```python
from build123d import *

# Parameters (mm, degrees)
F2_W     = 20
F2_H     = 20
F3_DEPTH = 2
F4_W     = 20
F4_H     = 20
F5_DEPTH = 18
F6_R     = 1.85
F7_DEPTH = 10


with BuildPart() as f3:
    # F2 (on Top) → F3 (new body)
    with BuildSketch(Plane.XY):
        with Locations((10, -10)):
            Rectangle(F2_W, F2_H)
    extrude(amount=F3_DEPTH)

    # F4 (on face) → F5 (join)
    with BuildSketch(Plane.XY.offset(2)):
        with Locations((10, -10)):
            Rectangle(F4_W, F4_H)
        Polygon((2, -6.06223871), (2, -2), (6.06223871, -2), (13.93776129, -2), (18, -2), (18, -6.06223871), (18, -13.93776129), (18, -18), (13.93776129, -18), (6.06223871, -18), (2, -18), (2, -13.93776129), align=None, mode=Mode.SUBTRACT)
        Polygon((6.06223871, -2), (2, -2), (2, -6.06223871), align=None)
        Polygon((18, -2), (13.93776129, -2), (18, -6.06223871), align=None)
        Polygon((18, -18), (18, -13.93776129), (13.93776129, -18), align=None)
        Polygon((6.06223871, -18), (2, -13.93776129), (2, -18), align=None)
    extrude(amount=F5_DEPTH)

    # F6 (on face) → F7 (cut)
    with BuildSketch(Plane.XY.offset(20)):
        with Locations((2.1344347065, -2.3655652935)):
            Circle(F6_R)
        with Locations((17.6344347065, -2.3655652935)):
            Circle(F6_R)
        with Locations((17.6344347065, -17.3655652935)):
            Circle(F6_R)
        with Locations((2.1344347065, -17.3655652935)):
            Circle(F6_R)
    extrude(amount=-F7_DEPTH, mode=Mode.SUBTRACT)


solid = f3.part
```
The listing builds one solid part. Answer for the finished solid, in the listing's coordinates (mm). A direction names the side the tool comes from. Round coordinates to 2 decimals unless told otherwise and drop trailing zeros. Loops run counter-clockwise (first coordinate to the right, second up) from the corner with the lowest first, then second, coordinate; pieces in that order, holes last. Notation, with made-up numbers: (39.5, 8) - (46.5, 8) arc R33 cw to (46.5, 39) - close; hole circle Ø7 at (-22.5, 39.25). An arc over 180 degrees is marked (long way). Return JSON: item names as keys, results as strings. Group by question number.
1. The part is cut by section C-C on z = 12.5. Determine the outline of the cut face in (x, y).
2. Consider probe 1 along X at (y, z) = (-7.25, 7.5); probe 2 along Y at (x, z) = (8.5, 11.5); probe 3 along Z at (x, y) = (8.75, -14.75). Determine where each line is inside the solid, lowest interval first.
3. Each of these flat-tipped pins is pushed along its axis until it touches: P1, Ø1.1, axis at x = 17, y = -2, coming from the +Z side; P2, Ø2, axis at x = 8, y = -8, coming from the +Z side. Where does it stop, or does it pass through?
4. The part is cut by section B-B on y = -7.5. Determine the outline of the cut face in (x, z).
5. The part is cut by section A-A on z = 4.5. Determine the outline of the cut face in (x, y), then the cut area to 3 significant figures.
6. The part is cut by section D-D on x = 13. Determine the outline of the cut face in (y, z), then the cut area to 3 significant figures.
7. The mould has two halves that part along X. Classify faces 1 (the flat face through (10, 0, 10)), 2 (the flat face through (0, -10, 10)), 3 (the cylindrical face through (17.23, -19.17, 15.07)), 4 (the flat face through (10, -18, 11)): pulls with the +X half, pulls with the -X half, needs draft (parallel to the pull), parting line crosses it, or undercut.
8. Which of the six approach directions +Z, -Z, +X, -X, +Y, -Y give full straight-line access (tool end or side, diameter ignored) to faces 5 (the flat face through (2, -2, 10)), 6 (the flat face through (10, -20, 10))?
Resolved:
{
 "1": {"outline": "(0, -20) - (20, -20) - (20, 0) - (0, 0) - close; hole circle Ø3.7 at (2.13, -17.37); hole circle Ø3.7 at (2.13, -2.37); hole (2, -13.94) - (6.06, -18) - (13.94, -18) - (18, -13.94) - (18, -6.06) - (13.94, -2) - (6.06, -2) - (2, -6.06) - close; hole circle Ø3.7 at (17.63, -17.37); hole circle Ø3.7 at (17.63, -2.37)"},
 "2": {"probe 1": "x = 0 to 2, 18 to 20", "probe 2": "y = -20 to -18, -2 to 0", "probe 3": "z = 0 to 2"},
 "3": {"P1": "stops at z = 10", "P2": "stops at z = 2"},
 "4": {"outline": "(0, 0) - (20, 0) - (20, 20) - (18, 20) - (18, 2) - (2, 2) - (2, 20) - (0, 20) - close"},
 "5": {"outline": "(0, -20) - (20, -20) - (20, 0) - (0, 0) - close; hole (2, -13.94) - (6.06, -18) - (13.94, -18) - (18, -13.94) - (18, -6.06) - (13.94, -2) - (6.06, -2) - (2, -6.06) - close", "area": "177 mm²"},
 "6": {"outline": "(-20, 0) - (0, 0) - (0, 20) - (-2, 20) - (-2, 2) - (-18, 2) - (-18, 20) - (-20, 20) - close", "area": "112 mm²"},
 "7": {"face 1": "needs draft", "face 2": "pulls with the -X half", "face 3": "undercut", "face 4": "undercut"},
 "8": {"face 5": "+Z", "face 6": "+Z, -Z, +X, -X, -Y"}
}
